from build123d import *

# Parameters (mm, degrees)
BOSS_EXTRUDE1_DEPTH     = 114.3
SKETCH3_R               = 10.16
BOSS_EXTRUDE2_DEPTH     = 20.32
SKETCH5_R               = 10.16
CUT_EXTRUDE1_DEPTH      = 12.7
FILLET2_R               = 2.54
SKETCH6_R               = 6.35
CUT_EXTRUDE2_DEPTH      = 129.953476168
BOSS_EXTRUDE3_START     = 43.791955851
BOSS_EXTRUDE3_DEPTH     = 3.198044249
BOSS_EXTRUDE3_START_2   = 49
BOSS_EXTRUDE3_2_DEPTH   = 17
CUT_EXTRUDE3_DEPTH      = 136.11033375
CUT_EXTRUDE3_DEPTH_BACK = 136.11033375
SKETCH8_W               = 15.239999981
SKETCH8_H               = 4.021184516
CUT_EXTRUDE4_DEPTH      = 135.882901337
CUT_EXTRUDE4_DEPTH_BACK = 135.882901337
SKETCH10_R              = 3.175
SKETCH11_R              = 5
CUT_EXTRUDE5_DEPTH      = 30


with BuildPart() as part:
    # Sketch2 → Boss-Extrude1 (new body)
    with BuildSketch(Plane.XY):
        with BuildLine():
            Line((-44.45, 0), (-32.512, 0))
            ThreePointArc((-32.512, 0), (0, 32.512), (32.512, 0))
            Line((32.512, 0), (44.45, 0))
            ThreePointArc((44.45, 0), (0, 44.45), (-44.45, 0))
        make_face()
    extrude(amount=BOSS_EXTRUDE1_DEPTH)

    # Sketch3 → Boss-Extrude2 (add)
    with BuildSketch(Plane.XZ):
        with Locations((44.45, 57.15)):
            Circle(SKETCH3_R)
        with Locations((-44.45, 57.15)):
            Circle(SKETCH3_R)
    extrude(amount=-BOSS_EXTRUDE2_DEPTH)

    # Sketch5 → Cut-Extrude1 (cut)
    with BuildSketch(Plane(origin=(0, 20.32, 0), x_dir=(1, 0, 0), z_dir=(0, 1, 0))):
        with Locations((44.45, -57.15)):
            Circle(SKETCH5_R)
        with Locations((-44.45, -57.15)):
            Circle(SKETCH5_R)
    extrude(amount=CUT_EXTRUDE1_DEPTH, mode=Mode.SUBTRACT)

    # Fillet2
    fillet2_edges = [part.edges().sort_by_distance(p)[0] for p in [
        (0, 44.45, 114.3),
        (0, 44.45, 0),
    ]]
    fillet(fillet2_edges, radius=FILLET2_R)

    # Sketch6 → Cut-Extrude2 (cut, through all)
    with BuildSketch(Plane(origin=(0, 20.32, 0), x_dir=(1, 0, 0), z_dir=(0, 1, 0))):
        with Locations(Location((44.45, -57.15, 0), (0, 0, 270))):
            Circle(SKETCH6_R)
        with Locations(Location((-44.45, -57.15, 0), (0, 0, 270))):
            Circle(SKETCH6_R)
    extrude(amount=-CUT_EXTRUDE2_DEPTH, mode=Mode.SUBTRACT)

    # Boss-Extrude3: read off the stored shape, not the designer's step
    # Boss-Extrude3 outline → Boss-Extrude3 (add)
    with BuildSketch(Plane(origin=(0, 0, 0), x_dir=(1, 0, 0), z_dir=(0, 1, 0)).offset(BOSS_EXTRUDE3_START)):
        with BuildLine():
            add(Edge.make_bspline(
                [(0, -49.53), (-1.008821651, -49.53), (-1.998619935, -49.72927394), (-3.843308667, -50.494879009), (-4.687454894, -51.060962916), (-6.791679377, -53.165741576), (-7.618847434, -55.15374527), (-7.620574374, -58.141520807), (-7.42290115, -59.141073642), (-6.658087545, -60.988450986), (-6.098856032, -61.827039285), (-4.680577167, -63.2461413), (-3.842032005, -63.805727128), (-1.998902378, -64.570532515), (-0.998499986, -64.769608068), (1.988013472, -64.770782097), (3.977148932, -63.946590903), (6.086279789, -61.841304586), (6.651483441, -61.000012912), (7.419760337, -59.152994739), (7.619200893, -58.162953427), (7.620794336, -56.149105114), (7.421964798, -55.156604804), (6.658890114, -53.313547431), (6.092840739, -52.467609132), (3.99113944, -50.362690075), (2.017643301, -49.53), (0, -49.53)],
                knots=[0, 0, 0, 0, 0.0625, 0.0625, 0.125, 0.125, 0.25, 0.25, 0.3125, 0.3125, 0.375, 0.375, 0.4375, 0.4375, 0.5, 0.5, 0.625, 0.625, 0.6875, 0.6875, 0.75, 0.75, 0.8125, 0.8125, 0.875, 0.875, 1, 1, 1, 1], degree=3))
        make_face()
    extrude(amount=BOSS_EXTRUDE3_DEPTH)

    # Boss-Extrude3 2 outline → Boss-Extrude3 2 (cut)
    with BuildSketch(Plane.XY.offset(BOSS_EXTRUDE3_START_2)):
        with BuildLine():
            Line((-9, 46.09176164), (-7.623050959, 46.33145572))
            ThreePointArc((-7.623050959, 46.33145572), (-3.825721713, 46.825057902), (0, 46.99))
            Line((0, 46.99), (-9, 46.9900001))
            Line((-9, 46.9900001), (-9, 46.09176164))
        make_face()
        with BuildLine():
            Line((9, 46.9900001), (0, 46.99))
            ThreePointArc((0, 46.99), (3.825781455, 46.825052741), (7.623169112, 46.331435152))
            Line((7.623169112, 46.331435152), (9, 46.091757812))
            Line((9, 46.091757812), (9, 46.9900001))
        make_face()
    extrude(amount=BOSS_EXTRUDE3_2_DEPTH, mode=Mode.SUBTRACT)

    # Sketch8 → Cut-Extrude3 (cut, two sides: drawn at the far end of the back side and taken through both)
    with BuildSketch(Plane.XY.offset(114.3).offset(-CUT_EXTRUDE3_DEPTH_BACK)):
        with Locations((9e-09, 48.342600124)):
            Rectangle(SKETCH8_W, SKETCH8_H)
    extrude(amount=CUT_EXTRUDE3_DEPTH + CUT_EXTRUDE3_DEPTH_BACK, mode=Mode.SUBTRACT)

    # Sketch10 → Cut-Extrude4 (cut, two sides: drawn at the far end of the back side and taken through both)
    with BuildSketch(Plane(origin=(0, 46.332007866, 0), x_dir=(1, 0, 0), z_dir=(0, 1, 0)).offset(-CUT_EXTRUDE4_DEPTH_BACK)):
        with Locations(Location((0, -57.15, 0), (0, 0, 270))):
            Circle(SKETCH10_R)
    extrude(amount=CUT_EXTRUDE4_DEPTH + CUT_EXTRUDE4_DEPTH_BACK, mode=Mode.SUBTRACT)

    # Sketch11 → Cut-Extrude5 (cut)
    with BuildSketch(Plane(origin=(0, 46.332007866, 0), x_dir=(1, 0, 0), z_dir=(0, 1, 0))):
        with Locations(Location((0, -57.15, 0), (0, 0, 270))):
            Circle(SKETCH11_R)
    extrude(amount=-CUT_EXTRUDE5_DEPTH, mode=Mode.SUBTRACT)


solid = part.part
Work out the finished part from the listing and answer in its coordinate system (mm). A direction names the side the tool comes from. Round coordinates to 2 decimals unless told otherwise and drop trailing zeros. Write each loop counter-clockwise with the first axis right and the second up, starting at its lowest first coordinate (ties: lowest second). Pieces come first, ordered by that corner, then holes.
1) A tool of negligible diameter and unlimited length cuts with its end or side. For faces 1 (the cylindrical face through (0.98, 44.44, 44.25)), 2 (the flat face through (49, 20.32, 62)), 3 (the flat face through (-40, 20.32, 62)), from which of +Z, -Z, +X, -X, +Y, -Y can it reach the whole face along a straight path? Write none if from no direction.
2) Given pin 1 Ø2 at (y, z) = (18, 97) entering from -X; pin 2 Ø5 at (x, z) = (0.5, 26.5) entering from -Y; pin 3 Ø22.5 at (x, z) = (41.5, 53.5) entering from +Y, each flat-ended and moving along its own axis, determine where each tip first touches the part or whether it passes through.
3) The mould has two halves that part along X. Classify faces 4 (the cylindrical face through (-34.29, 23.36, 57.3)), 5 (the cylindrical face through (34.29, 23.36, 57)), 6 (the cylindrical face through (-40.16, 10.3, 52.47)), 7 (the flat face through (36, 0, 58)): pulls with the +X half, pulls with the -X half, needs draft (parallel to the pull), parting line crosses it, or undercut.
4) A cutting plane is placed at A-A (y = 10). Give the number of separate pieces and of enclosed holes in the cut face, plus the area to 3 significant figures.
5) Straight lines are drawn through the part: line 1 (Z direction, x = 0, y = 40.75); line 2 (Z direction, x = 44, y = 10); line 3 (X direction, y = 5, z = 57.15). For each, find the intervals that lie inside material, in ascending order.
6) A cutting plane is placed at B-B (z = 87.5). Give the vertices of the cut face in (x, y), plus the area to 3 significant figures.
Completed:
1. face 1: +Y
1. face 2: +X, +Y
1. face 3: -X, +Y
2. pin 1: stops at x = -41.07
2. pin 2: stops at y = 32.37
2. pin 3: stops at y = 32.57
3. face 4: pulls with the -X half
3. face 5: pulls with the +X half
3. face 6: undercut
3. face 7: needs draft
4. separate pieces: 2
4. enclosed holes: 2
4. area: 2,940 mm2
5. line 1: z = 0 to 52.15, 62.15 to 114.3
5. line 2: z = 47 to 50.82, 63.48 to 67.3
5. line 3: x = -54.61 to -50.8, -38.1 to -32.13, 32.13 to 38.1, 50.8 to 54.61
6. outline: (-44.45, 0) - (-32.51, 0) arc R32.51 cw to (32.51, 0) - (44.45, 0) arc R44.45 ccw to start
6. area: 1,440 mm2
